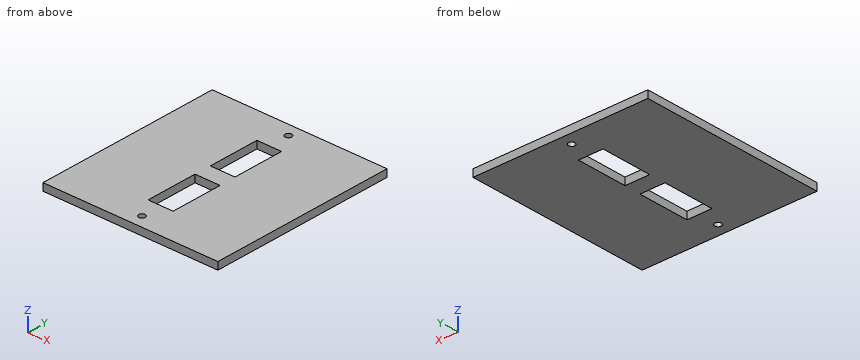
```python
from build123d import *

# Parameters (mm, degrees)
SKETCH1_W           = 75.17
SKETCH1_H           = 80.17
SKETCH1_W_2         = 10.75
SKETCH1_H_2         = 22.25
SKETCH1_W_3         = 10.58
SKETCH1_H_3         = 22.08
BOSS_EXTRUDE1_DEPTH = 3.175
SKETCH2_R           = 1.415
CUT_EXTRUDE1_DEPTH  = 4.175


with BuildPart() as part:
    # Sketch1 → Boss-Extrude1 (new body)
    with BuildSketch(Plane.XY):
        Rectangle(SKETCH1_W, SKETCH1_H)
        with Locations((0, -14.675)):
            Rectangle(SKETCH1_W_2, SKETCH1_H_2, mode=Mode.SUBTRACT)
        with Locations((0, 14.675)):
            Rectangle(SKETCH1_W_3, SKETCH1_H_3, mode=Mode.SUBTRACT)
    extrude(amount=BOSS_EXTRUDE1_DEPTH)

    # Sketch2 → Cut-Extrude1 (cut, through all)
    with BuildSketch(Plane.XY.offset(3.175)):
        with Locations((0.085, 34.696699141)):
            Circle(SKETCH2_R)
        with Locations((0.085, -34.696699141)):
            Circle(SKETCH2_R)
    extrude(amount=-CUT_EXTRUDE1_DEPTH, mode=Mode.SUBTRACT)


solid = part.part
```
Read the model definition and answer for the solid it produces. Units are mm, in the model's axes. Give positions to 0.01 mm unless a question says otherwise; leave off trailing zeros. Loops run counter-clockwise (first coordinate to the right, second up) from the corner with the lowest first, then second, coordinate; pieces in that order, holes last.
Item 1: The part is cut by section C-C (z = 2). Write down the section's boundary in (x, y) (3 decimals).
Item 2: This flat-tipped pin is pushed along its axis until it touches: pin 1 Ø2.5 at (x, y) = (0.08, -34.7) entering from +Z. Where does it stop, or does it pass through?
Item 3: The part is cut by section A-A (x = -4). Write down the section's boundary in (y, z) (3 decimals), and give its area (3 significant figures).
Item 4: Find the intervals of material crossed by line 1 along X through (y, z) = (7, 0.25) (3 decimals); line 2 along Y through (x, z) = (0, 1.7) (3 decimals); line 3 along Y through (x, z) = (2.5, 2.2) (3 decimals), in increasing order.
Item 5: The part is cut by section B-B (y = 13). Write down the section's boundary in (x, z) (3 decimals).
Taken from the geometry:
1. outline: (-37.585, -40.085) - (37.585, -40.085) - (37.585, 40.085) - (-37.585, 40.085) - close; hole (-5.375, -25.8) - (5.375, -25.8) - (5.375, -3.55) - (-5.375, -3.55) - close; hole (-5.29, 3.635) - (5.29, 3.635) - (5.29, 25.715) - (-5.29, 25.715) - close; hole circle Ø2.83 at (0.085, -34.697); hole circle Ø2.83 at (0.085, 34.697)
2. pin 1: passes through
3. outline: (-40.085, 0) - (-25.8, 0) - (-25.8, 3.175) - (-40.085, 3.175) - close; (-3.55, 0) - (3.635, 0) - (3.635, 3.175) - (-3.55, 3.175) - close; (25.715, 0) - (40.085, 0) - (40.085, 3.175) - (25.715, 3.175) - close
3. area: 114 mm2
4. line 1: x = -37.585 to -5.29, 5.29 to 37.585
4. line 2: y = -40.085 to -36.109, -33.284 to -25.8, -3.55 to 3.635, 25.715 to 33.284, 36.109 to 40.085
4. line 3: y = -40.085 to -25.8, -3.55 to 3.635, 25.715 to 40.085
5. outline: (-37.585, 0) - (-5.29, 0) - (-5.29, 3.175) - (-37.585, 3.175) - close; (5.29, 0) - (37.585, 0) - (37.585, 3.175) - (5.29, 3.175) - close
